Autodesk Inventor part; units mm, degrees
ref_plane "YZ Plane" through (0, 0, 0) normal (1, 0, 0) x (0, 1, 0)
ref_plane "XZ Plane" through (0, 0, 0) normal (0, 1, 0) x (-1, 0, 0)
ref_plane "XY Plane" through (0, 0, 0) normal (0, 0, 1) x (1, 0, 0)
sketch "Sketch1" plane through (0, 0, 0) normal (0, 0, 1) x (1, 0, 0)
  line L0 (-67.5, -22.5) -> (67.5, -22.5)
  line L1 (67.5, -22.5) -> (67.5, 22.5)
  line L2 (67.5, 22.5) -> (-67.5, 22.5)
  line L3 (-67.5, 22.5) -> (-67.5, -22.5)
  line L4 (-67.5, -22.5) -> (67.5, 22.5) construction
  line L5 (67.5, -22.5) -> (-67.5, 22.5) construction
  line L6 (0, -5) -> (0, 5) construction
  line L7 (-3, -5) -> (-3, 5)
  line L8 (3, 5) -> (3, -5)
  arc A0 (-3, -5) -> (3, -5) centre (0, -5) ccw
  arc A1 (3, 5) -> (-3, 5) centre (0, 5) ccw
  line L9 (0, 0) -> (67.5, 0)
  circle A2 centre (52, 19) radius 1.6
  line L10 (-20, 26) -> (20, 26)
  line L11 (20, 26) -> (20, 22.5)
  line L12 (20, 22.5) -> (-20, 22.5)
  line L13 (-20, 22.5) -> (-20, 26)
  line L14 (-20, 26) -> (20, 22.5) construction
  line L15 (20, 26) -> (-20, 22.5) construction
  line L16 (-20, -26) -> (20, -26)
  line L17 (20, -26) -> (20, -22.5)
  line L18 (20, -22.5) -> (-20, -22.5)
  line L19 (-20, -22.5) -> (-20, -26)
  line L20 (-20, -26) -> (20, -22.5) construction
  line L21 (20, -26) -> (-20, -22.5) construction
  circle A3 centre (52, -19) radius 1.6
  point P0 (0, -8)
  point P1 (0, 8)
  point P2 (0, 24.25)
  point P3 (0, 22.5)
  point P4 (0, 22.5)
  point P5 (0, -24.25)
  point P6 (0, -22.5)
  point P7 (0, -22.5)
  dimension "d0" = 135
  dimension "d1" = 45
  dimension "d13" = 16
  dimension "d14" = 3
  dimension "d15" = 3.2
  dimension "d16" = 55
  dimension "d17" = 38
  dimension "d18" = 40
  dimension "d19" = 3.5
sketch "Sketch2" plane through (0, 0, 1.5) normal (0, 0, 1) x (1, 0, 0)
  line L0 (67.5, -22.5) -> (67.5, 22.5)
  line L1 (67.5, -22.5) -> (92.5, -55)
  line L2 (67.5, 0) -> (0, 0)
  line L3 (67.5, 22.5) -> (92.5, 55)
  line L4 (92.5, 55) -> (92.5, -55)
  dimension "d20" = 25
  dimension "d21" = 110
extrude "Plate1" add sketch "Sketch1" along normal mid plane 3
sheet face with bend "Face2" sketch "Sketch2" thickness 3 toward (0, 0, -1) bend radius 3
bend "Bend1"
equation "\"d9\" = Thickness"
equation "\"d22\" = BendRadius"
equation "\"d23\" = BendReliefWidth"
equation "\"d25\" = MinimumRemnant"
equation "\"d24\" = BendReliefDepth"
equation "\"d26\" = TransitionRadius"
equation "\"BendRadius\" = Thickness"
equation "\"BendReliefWidth\" = Thickness"
equation "\"BendReliefDepth\" = 0.5 * Thickness"
equation "\"CornerReliefSize\" = 4 * Thickness"
equation "\"MinimumRemnant\" = 2 * Thickness"
equation "\"TransitionRadius\" = BendRadius"
equation "\"JacobiRadiusSize\" = BendRadius"
equation "\"GapSize\" = Thickness"
properties part number "Path"
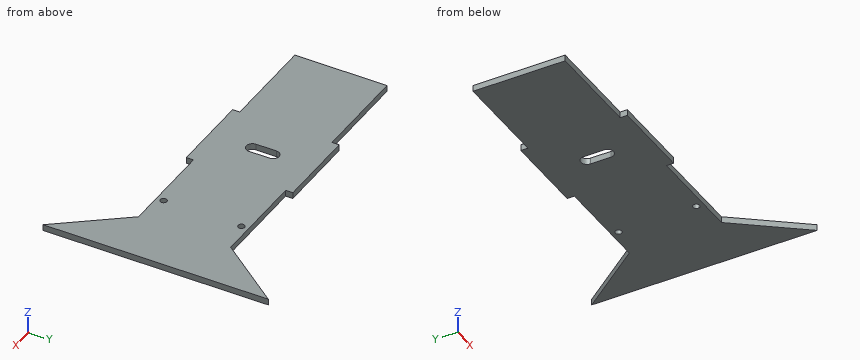
Work out the finished part from the listing and answer in its coordinate system (mm). Give positions to 0.01 mm unless a question says otherwise; leave off trailing zeros. Write each loop counter-clockwise with the first axis right and the second up, starting at its lowest first coordinate (ties: lowest second). Pieces come first, ordered by that corner, then holes. Notation, with made-up numbers: (-5.5, 14.5) - (47.5, 14.5) arc R23 cw to (47.5, 47.5) - close; hole circle Ø7 at (-28, -27.75). An arc over 180 degrees is marked (long way). One line per item, written item: value. Start each with the question number.
1. Given pin 1 (0.9 mm diameter, centred on x = -8, z = 0.5, fed in from -Y); pin 2 (0.9 mm diameter, centred on x = 36, z = -0.5, fed in from -Y); pin 3 (0.9 mm diameter, centred on x = -46.5, z = 0, fed in from +Y), each flat-ended and moving along its own axis, determine where each tip first touches the part or whether it passes through.
2. Find section B-B (x = 0). Write down the section's boundary in (y, z), then the cut area to 3 significant figures.
3. Consider probe 1 along Y at (x, z) = (52, 0.8); probe 2 along Y at (x, z) = (-19.5, -0.95); probe 3 along Y at (x, z) = (52.5, 0). Determine where each line is inside the solid, lowest interval first.
4. Find section D-D (x = 52). Write down the section's boundary in (y, z).
5. Find section C-C (z = 0.5). Write down the section's boundary in (x, y).
6. Find section A-A (y = 1.5). Write down the section's boundary in (x, z), then the cut area to 3 significant figures.
Geometry results:
1. pin 1: y = -26
1. pin 2: y = -22.5
1. pin 3: y = 22.5
2. outline: (-26, -1.5) - (-8, -1.5) - (-8, 1.5) - (-26, 1.5) - close; (8, -1.5) - (26, -1.5) - (26, 1.5) - (8, 1.5) - close
2. area: 108 mm2
3. probe 1: -22.5 to -20.6, -17.4 to 17.4, 20.6 to 22.5
3. probe 2: -26 to 26
3. probe 3: -22.5 to -20.52, -17.48 to 17.48, 20.52 to 22.5
4. outline: (-22.5, -1.5) - (-20.6, -1.5) - (-20.6, 1.5) - (-22.5, 1.5) - close; (-17.4, -1.5) - (17.4, -1.5) - (17.4, 1.5) - (-17.4, 1.5) - close; (20.6, -1.5) - (22.5, -1.5) - (22.5, 1.5) - (20.6, 1.5) - close
5. outline: (-67.5, -22.5) - (-20, -22.5) - (-20, -26) - (20, -26) - (20, -22.5) - (67.5, -22.5) - (92.5, -55) - (92.5, 55) - (67.5, 22.5) - (20, 22.5) - (20, 26) - (-20, 26) - (-20, 22.5) - (-67.5, 22.5) - close; hole (-3, -5) arc R3 ccw to (3, -5) - (3, 5) arc R3 ccw to (-3, 5) - close; hole circle Ø3.2 at (52, -19); hole circle Ø3.2 at (52, 19)
6. outline: (-67.5, -1.5) - (-3, -1.5) - (-3, 1.5) - (-67.5, 1.5) - close; (3, -1.5) - (92.5, -1.5) - (92.5, 1.5) - (3, 1.5) - close
6. area: 462 mm2
